Build history of the part. All positions in model axes, mm. A direction names the side the tool comes from. Coordinates: 2 decimals unless noted, no trailing zeros. Loops run counter-clockwise (first coordinate to the right, second up) from the corner with the lowest first, then second, coordinate; pieces in that order, holes last.
Item 1: Cut at B-B (x = 27.5). List the corners of the cut face in (y, z) (3 decimals).
Item 2: 3-axis set-ups, long thin cutter, end or side, ignore diameter. For faces 1 (the face through (-3.131, 3.441, -15.497)), 2 (the face through (31.18, 9.085, 2.861)): which of +Z, -Z, +X, -X, +Y, -Y reach the whole face in a straight line?
Item 3: Cut at D-D (z = 10.5). List the corners of the cut face in (x, y).
Item 4: Mould opens along X. For faces 3 (the face through (60.443, -4.696, 0.717)), 4 (the face through (0, -7, -7)), 5 (the face through (58, 0, 0)), 6 (the face through (-6.35, 0, 0)) say: released by +X, released by -X, zero draft, split by the parting line, or undercut.
Item 5: Cut at A-A (z = 0). List the corners of the cut face in (x, y) (3 decimals), and give its area (3 significant figures).
Item 6: Drill centre lines: line 1 along X through (y, z) = (-4.5, 0); line 2 along X through (y, z) = (-8, -2.5); line 3 along X through (y, z) = (0.5, 13.5). Where is each one in solid material? Low to high.
Item 7: Flat gauge pins, fed straight in: pin 1 (6 mm diameter, centred on x = 35, y = -9, fed in from -Z); pin 2 (1 mm diameter, centred on x = 19.5, z = 12, fed in from +Y); pin 3 (2 mm diameter, centred on y = -11.5, z = 2, fed in from +X); pin 4 (4 mm diameter, centred on x = 58.5, z = -0.5, fed in from -Y). Where does each tip first touch, or does it go through?
Item 8: Cut at C-C (y = -12.5). List the corners of the cut face in (x, z).
from build123d import *

# Parameters (mm, degrees)
F0_R     = 9.525
F1_DEPTH = 64.516
F3_R     = 15.875
F4_DEPTH = 6.35
F2_R     = 2.3876
F5_DEPTH = 15.876
F6_R     = 1.27


with BuildPart() as f1:
    # F0 (on Right) → F1 (new body)
    with BuildSketch(Plane.YZ):
        Circle(F0_R)
    extrude(amount=F1_DEPTH)

    # F3 (on face) → F4 (join)
    with BuildSketch(Plane(origin=(0, 0, 0), x_dir=(0, -1, 0), z_dir=(-1, 0, 0))):
        Circle(F3_R)
    extrude(amount=F4_DEPTH)

    # F2 (on Front) → F5 (cut, through all)
    with BuildSketch(Plane.XZ):
        with Locations((58.166, 0)):
            Circle(F2_R)
    extrude(amount=F5_DEPTH, mode=Mode.SUBTRACT)

    # F6
    f6_edges = [f1.edges().sort_by_distance(p)[0] for p in [
        (64.516, -9.525, 0),
    ]]
    fillet(f6_edges, radius=F6_R)


solid = f1.part
Filled sheet:
1. outline: circle Ø19.05 at (0, 0)
2. face 1: +X, -X
2. face 2: +X
3. outline: (-6.35, -11.91) - (0, -11.91) - (0, 11.91) - (-6.35, 11.91) - close
4. face 3: undercut
4. face 4: released by +X
4. face 5: undercut
4. face 6: released by -X
5. outline: (-6.35, -15.875) - (0, -15.875) - (0, -9.525) - (55.778, -9.525) - (55.778, 0) - (60.554, 0) - (60.554, -9.525) - (63.246, -9.525) arc R1.27 ccw to (64.516, -8.255) - (64.516, 8.255) arc R1.27 ccw to (63.246, 9.525) - (0, 9.525) - (0, 15.875) - (-6.35, 15.875) - close
5. area: 1,380 mm2
6. line 1: x = -6.35 to 55.78, 60.55 to 64.52
6. line 2: x = -6.35 to 64.51
6. line 3: x = -6.35 to 0
7. pin 1: stops at z = -7.4
7. pin 2: passes through
7. pin 3: stops at x = 0
7. pin 4: stops at y = -9.51
8. outline: (-6.35, -9.79) - (0, -9.79) - (0, 9.79) - (-6.35, 9.79) - close
